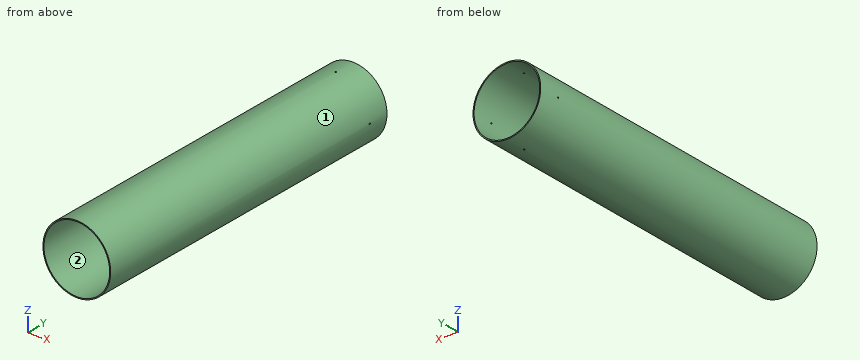
from build123d import *

# Parameters (mm, degrees)
SKETCH1_R           = 51.1048
SKETCH1_R_2         = 49.53
BOSS_EXTRUDE1_DEPTH = 508
SKETCH2_R           = 1.0922
CUT_EXTRUDE1_DEPTH  = 52.1048
CIRPATTERN2_COUNT   = 4


with BuildPart() as part:
    # Sketch1 → Boss-Extrude1 (new body)
    with BuildSketch(Plane(origin=(0, 0, 0), x_dir=(1, 0, 0), z_dir=(0, 1, 0))):
        Circle(SKETCH1_R)
        Circle(SKETCH1_R_2, mode=Mode.SUBTRACT)
    extrude(amount=BOSS_EXTRUDE1_DEPTH)

    # Sketch2 → Cut-Extrude1 (cut, through all)
    with BuildSketch(Plane.XY):
        with Locations((0, 476.25)):
            Circle(SKETCH2_R)
    cut_extrude1 = extrude(amount=-CUT_EXTRUDE1_DEPTH, mode=Mode.SUBTRACT)

    # CirPattern2: Cut-Extrude1 ×4 about axis
    cirpattern2_axis = Axis((0, 508, 0), (0, -1, 0))
    for i in range(1, CIRPATTERN2_COUNT):
        add(cut_extrude1.rotate(cirpattern2_axis, i * 360 / CIRPATTERN2_COUNT), mode=Mode.SUBTRACT)


solid = part.part
The model under review builds one solid part; all positions refer to its coordinate system, in mm. Face numbers are marked on the shaded views. Give positions to 0.01 mm unless a question says otherwise; leave off trailing zeros. Loops run counter-clockwise (first coordinate to the right, second up) from the corner with the lowest first, then second, coordinate; pieces in that order, holes last. Notation, with made-up numbers: (71.25, -10) -> (76.25, -10) arc R22 ccw to (76.25, 19) -> close; hole circle Ø5 at (82.25, 83.5). An arc over 180 degrees is marked (long way). Answer as a JSON object with one key per item and string values. Group by question number.
Q1. Take a section at B-B (z = 17). Write out the cut boundary in (x, y).
Q2. Take a section at C-C (y = 398.5). Write out the cut boundary in (x, z), plus the area to 3 significant figures.
Q3. Wall thickness on line 1 along X through (y, z) = (326, 2.5); line 2 along X through (y, z) = (377, 0); line 3 along Y through (x, z) = (0, -50): over which ranges is each line inside the solid? List them lowest first.
Q4. Take a section at A-A (x = -19.5). Write out the cut boundary in (y, z).
Q5. Insertion check: pin 1 (5 mm diameter, centred on y = 211.5, z = 14.5, fed in from -X); pin 2 (2.5 mm diameter, centred on y = 476.25, z = 0, fed in from -X); pin 3 (1 mm diameter, centred on y = 265.5, z = -17, fed in from +X); pin 4 (8 mm diameter, centred on x = 20, y = 203.5, fed in from +Z). Each pin has a flat end and moves straight along its axis. Give the tip position at first contact, or say it passes through.
Q6. Draft analysis for pull direction X (two halves, no side actions). For the marked faces 1 and 2, state which applies: pulls with the +X half, pulls with the -X half, needs draft (parallel to the pull), parting line crosses it, or undercut.
Answer below:
{
 "1": {"outline": "(-48.19, 0) -> (-46.52, 0) -> (-46.52, 508) -> (-48.19, 508) -> close; (46.52, 0) -> (48.19, 0) -> (48.19, 508) -> (46.52, 508) -> close"},
 "2": {"outline": "circle Ø102.21 at (0, 0); hole circle Ø99.06 at (0, 0)", "area": "498 mm2"},
 "3": {"line 1": "x = -51.04 to -49.47, 49.47 to 51.04", "line 2": "x = -51.1 to -49.53, 49.53 to 51.1", "line 3": "y = 0 to 475.16, 477.34 to 508"},
 "4": {"outline": "(0, -47.24) -> (508, -47.24) -> (508, -45.53) -> (0, -45.53) -> close; (0, 45.53) -> (508, 45.53) -> (508, 47.24) -> (0, 47.24) -> close"},
 "5": {"pin 1": "stops at x = -49.68", "pin 2": "stops at x = -51.1", "pin 3": "stops at x = 48.37", "pin 4": "stops at z = 48.54"},
 "6": {"face 1": "parting line crosses it", "face 2": "undercut"}
}
